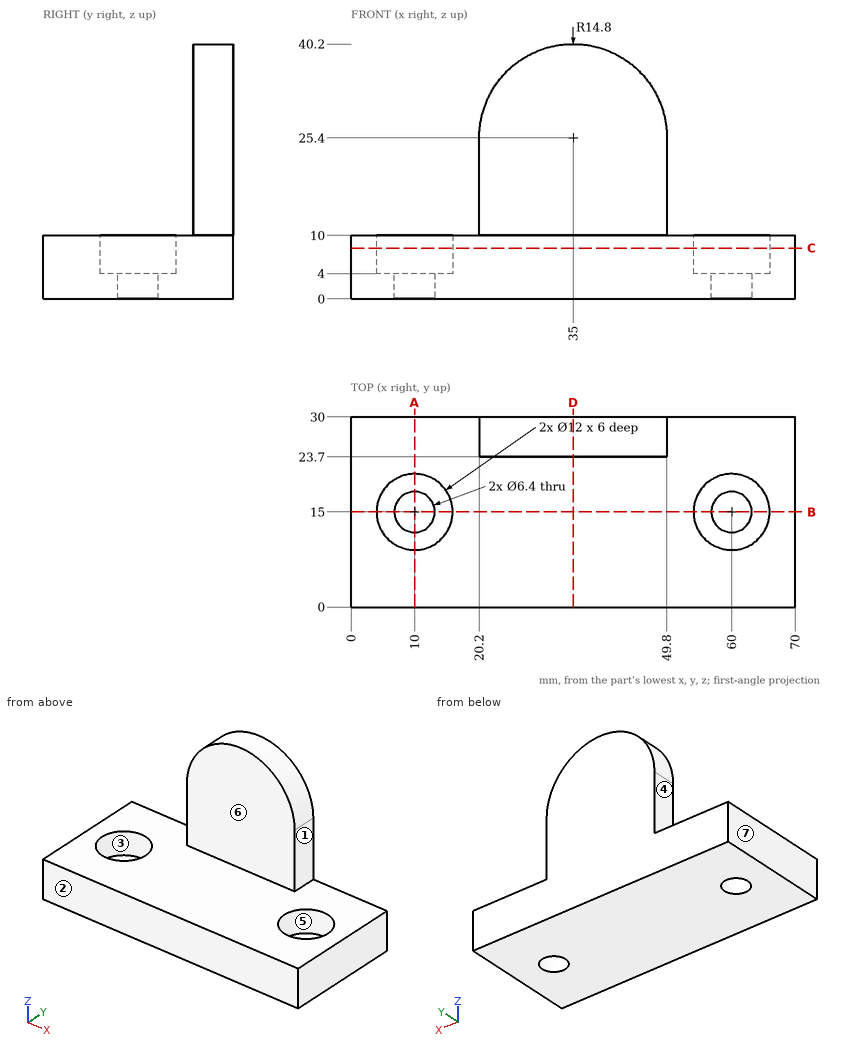
Can you work these out from the drawing? Everything is in mm from the part's minimum corner. A direction names the side the tool comes from. Coordinates: 2 decimals unless noted, no trailing zeros. Loops run counter-clockwise (first coordinate to the right, second up) from the corner with the lowest first, then second, coordinate; pieces in that order, holes last. Notation, with made-up numbers: (5, 52) -> (49, 52) arc R33 ccw to (49, 88) -> close; hole circle Ø5 at (-7.5, -36). An arc over 180 degrees is marked (long way). Return JSON: item names as keys, results as strings.
1) I need wall thicknesses on line 1 (Y direction, x = 10, z = 8); line 2 (Z direction, x = 48.5, y = 4); line 3 (Y direction, x = 60, z = 2.55). Which ranges of each line are inside material? Lowest first, please. Write a range as from..to.
Results below:
{"line 1": "0..9, 21..30", "line 2": "0..10", "line 3": "0..11.8, 18.2..30"}
2) If we section it at B-B, the plane y = 15: Write out the boundary of the cut face in (x, z), then the cut area to 3 significant figures.
Results below:
{"outline": "(0, 0) -> (6.8, 0) -> (6.8, 4) -> (4, 4) -> (4, 10) -> (0, 10) -> close; (13.2, 0) -> (56.8, 0) -> (56.8, 4) -> (54, 4) -> (54, 10) -> (16, 10) -> (16, 4) -> (13.2, 4) -> close; (63.2, 0) -> (70, 0) -> (70, 10) -> (66, 10) -> (66, 4) -> (63.2, 4) -> close", "area": "505 mm²"}
3) Thinking about a two-plate mould opening in Y: for the marked faces 1, 2 and 3, which applies, +Y half, -Y half, draft (parallel to the pull), parting line (faces both ways), or undercut?
Results below:
{"face 1": "draft", "face 2": "-Y half", "face 3": "undercut"}
4) If we section it at C-C, the plane z = 8: Write out the boundary of the cut face in (x, y).
Results below:
{"outline": "(0, 0) -> (70, 0) -> (70, 30) -> (0, 30) -> close; hole circle Ø12 at (10, 15); hole circle Ø12 at (60, 15)"}
5) If we section it at D-D, the plane x = 35: Write out the boundary of the cut face in (y, z), then the cut area to 3 significant figures.
Results below:
{"outline": "(0, 0) -> (30, 0) -> (30, 40.2) -> (23.7, 40.2) -> (23.7, 10) -> (0, 10) -> close", "area": "490 mm²"}
6) If we section it at A-A, the plane x = 10: Write out the boundary of the cut face in (y, z), then the cut area to 3 significant figures.
Results below:
{"outline": "(0, 0) -> (11.8, 0) -> (11.8, 4) -> (9, 4) -> (9, 10) -> (0, 10) -> close; (18.2, 0) -> (30, 0) -> (30, 10) -> (21, 10) -> (21, 4) -> (18.2, 4) -> close", "area": "202 mm²"}
7) For the marked faces 4, 5, 6 and 7, which set-ups out of +Z, -Z, +X, -X, +Y, -Y let a thin tool reach every point of the face, with its end or its side?
Results below:
{"face 4": "+Z, -X, +Y, -Y", "face 5": "+Z", "face 6": "+Z, +X, -X, -Y", "face 7": "+Z, -Z, -X, +Y, -Y"}
8) Will these pins go through, and if not, where does the flat tip stop? pin 1 (12 mm diameter, centred on y = 20.5, z = 32.5, fed in from -X); pin 2 (10 mm diameter, centred on x = 15.5, z = 27.5, fed in from -Y); pin 3 (10 mm diameter, centred on x = 14.5, y = 20.5, fed in from +Z).
Results below:
{"pin 1": "x = 20.34", "pin 2": "y = 23.7", "pin 3": "z = 10"}
